Read the model definition and answer for the solid it produces. Units are mm, in the model's axes. Coordinates: 2 decimals unless noted, no trailing zeros. Order: outer loops, then holes, each group sorted by start corner. A loop starts at its lowest first (then second) coordinate and runs counter-clockwise, first axis right, second up. Notation, with made-up numbers: M 4,-29 L 37,-29 A20 ccw 37,-6 Z; hole C 31.5,56.5 d3. An arc over 180 degrees is marked long. One line per question, with ' | ' between items. Start each with the question number.
1) Consider probe 1 along X at (y, z) = (0.4, 7.62) (3 decimals); probe 2 along X at (y, z) = (1, 6) (3 decimals); probe 3 along Z at (x, y) = (6.5, 2.2). Determine where each line is inside the solid, lowest interval first.
2) Given P1, Ø6, axis at x = -5.715, z = 7.62, coming from the +Y side, flat-ended and moving along its own axis, determine where the tip first touches the part or whether it passes through.
3) Find section B-B, the plane y = 1.6. Write down the section's boundary in (x, z) (3 decimals), plus the area to 3 significant figures.
4) The mould has two halves that part along X. Classify faces 1 (the face through (0, 2, -11.43)), 2 (the face through (-6.316, 1.401, 9.529)), 3 (the face through (-14.605, 2, 0)), 4 (the face through (14.605, 2, 0)): +X half, -X half, draft (parallel to the pull), parting line (faces both ways), or undercut.
5) Find section A-A, the plane z = 7.62. Write down the section's boundary in (x, y) (3 decimals).
from build123d import *

# Parameters (mm, degrees)
SKETCH1_W                                     = 29.21
SKETCH1_H                                     = 22.86
BOSS_EXTRUDE1_DEPTH                           = 3.175
CSK_FOR_6_FLAT_HEAD_MACHINE_SCREW1_AT_2_COUNT = 2
CSK_FOR_6_FLAT_HEAD_MACHINE_SCREW1_AT_2_PITCH = 11.43


with BuildPart() as part:
    # Sketch1 → Boss-Extrude1 (new body)
    with BuildSketch(Plane(origin=(0, 0, 0), x_dir=(1, 0, 0), z_dir=(0, 1, 0))):
        Rectangle(SKETCH1_W, SKETCH1_H)
    extrude(amount=BOSS_EXTRUDE1_DEPTH)

    # Sketch5 → CSK for #6 Flat Head Machine Screw1 (revolve, cut)
    with BuildSketch(Plane(origin=(-5.715, 3.175, 7.62), x_dir=(0, 0, 1), z_dir=(1, 0, 0))):
        Polygon((0, 0), (0, 3.175), (1.89865, 3.175), (1.89865, 1.891953401), (3.5433, 0), align=None)
    csk_for_6_flat_head_machine_screw1 = revolve(axis=Axis((-5.715, 9.525, 7.62), (0, -1, 0)), mode=Mode.SUBTRACT)

    # CSK for #6 Flat Head Machine Screw1 at 2: CSK for #6 Flat Head Machine Screw1 ×2
    with Locations(*[(i * CSK_FOR_6_FLAT_HEAD_MACHINE_SCREW1_AT_2_PITCH, 0, 0) for i in range(1, CSK_FOR_6_FLAT_HEAD_MACHINE_SCREW1_AT_2_COUNT)]):
        add(csk_for_6_flat_head_machine_screw1, mode=Mode.SUBTRACT)


solid = part.part
Report:
1) probe 1: x = -14.605 to -7.614, -3.816 to 3.816, 7.614 to 14.605 | probe 2: x = -14.605 to -6.705, -4.725 to 4.725, 6.705 to 14.605 | probe 3: z = -11.43 to 5.04, 10.2 to 11.43
2) P1: stops at y = 2.55
3) outline: M -14.605,-11.43 L 14.605,-11.43 L 14.605,11.43 L -14.605,11.43 Z; hole C -5.715,7.62 d4.348; hole C 5.715,7.62 d4.348 | area: 638 mm^2
4) face 1: draft | face 2: undercut | face 3: -X half | face 4: +X half
5) outline: M -14.605,0 L -7.614,0 L -7.614,1.283 L -9.258,3.175 L -14.605,3.175 Z; M -3.816,0 L 3.816,0 L 3.816,1.283 L 2.172,3.175 L -2.172,3.175 L -3.816,1.283 Z; M 7.614,0 L 14.605,0 L 14.605,3.175 L 9.258,3.175 L 7.614,1.283 Z
